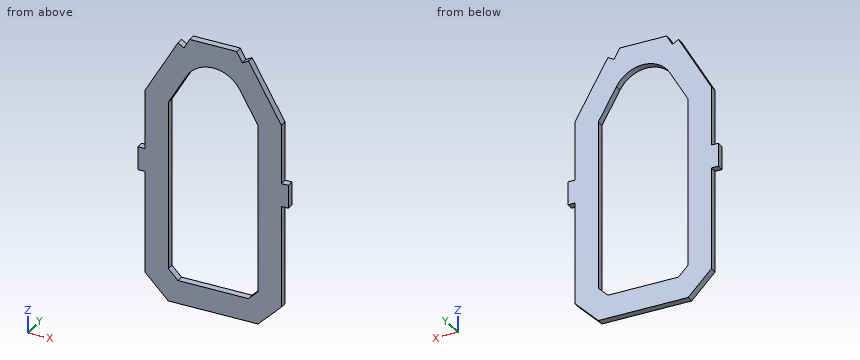
from build123d import *

# Parameters (mm, degrees)
F1_DEPTH = 1.5


with BuildPart() as f1:
    # F0 (on Front) → F1 (new body, symmetric)
    with BuildSketch(Plane.XZ):
        Polygon((-19.25, -59), (19.25, -59), (29.25, -49), (29.25, -5), (32.25, -5), (32.25, 5), (29.25, 5), (29.25, 30.43933), (15.1342262987, 54.8714219789), (12.5366059283, 53.370632716), (10.0352904902, 57.7), (-10.0352904902, 57.7), (-12.5366059283, 53.370632716), (-15.1342262987, 54.8714219789), (-29.25, 30.43933), (-29.25, 5), (-32.25, 5), (-32.25, -5), (-29.25, -5), (-29.25, -49), align=None)
        with BuildLine():
            Line((19.25, 0), (19.25, -44.8578643763))
            Line((19.25, -44.8578643763), (15.1078643763, -49))
            Line((15.1078643763, -49), (-15.1078643763, -49))
            Line((-15.1078643763, -49), (-19.25, -44.8578643763))
            Line((-19.25, -44.8578643763), (-19.25, 0))
            Line((-19.25, 0), (-19.25, 27.7582098748))
            Line((-19.25, 27.7582098748), (-11.4781226068, 41.2100565349))
            ThreePointArc((-11.4781226068, 41.2100565349), (-0.0096357275, 47.8457480828), (11.4684858529, 41.2267361773))
            Line((11.4684858529, 41.2267361773), (19.25, 27.7582098748))
            Line((19.25, 27.7582098748), (19.25, 0))
        make_face(mode=Mode.SUBTRACT)
    extrude(amount=F1_DEPTH, both=True)


solid = f1.part
Source: CAD feature listing. Evaluate the final solid. Frame: model axes, mm. Give positions to 0.01 mm unless a question says otherwise; leave off trailing zeros. Order: outer loops, then holes, each group sorted by start corner. A loop starts at its lowest first (then second) coordinate and runs counter-clockwise, first axis right, second up. Notation, with made-up numbers: (-24, 76) -> (-3, 76) arc R33 cw to (-3, 112) -> close; hole circle Ø8 at (-32.75, 61.5). An arc over 180 degrees is marked (long way). Write item = value, one per line.
Q1. Cut plane B-B, the plane x = -16.5. Output: boundary loops of the cut face in (y, z), and give its area (3 significant figures).
Data:
outline = (-1.5, -59) -> (1.5, -59) -> (1.5, -47.61) -> (-1.5, -47.61) -> close; (-1.5, 32.52) -> (1.5, 32.52) -> (1.5, 52.51) -> (-1.5, 52.51) -> close
area = 94.1 mm^2
Q2. Cut plane D-D, the plane x = -25.5. Output: boundary loops of the cut face in (y, z), and give its area (3 significant figures).
Data:
outline = (-1.5, -52.75) -> (1.5, -52.75) -> (1.5, 36.93) -> (-1.5, 36.93) -> close
area = 269 mm^2
Q3. Material intervals for line 1 (X direction, y = -0.95, z = -30.5); line 2 (Z direction, x = 4.5, y = -1.25); line 3 (Z direction, x = 29.5, y = -1), sorted ascending. Write a range as from..to.
Data:
line_1 = -29.25..-19.25, 19.25..29.25
line_2 = -59..-49, 47.06..57.7
line_3 = -5..5
Q4. Pin query (flat end, axial travel): pin 1 (1.5 mm diameter, centred on y = -0.5, z = 21.5, fed in from -X); pin 2 (1.5 mm diameter, centred on x = 30.5, y = -0.5, fed in from +Z); pin 3 (1.5 mm diameter, centred on x = 30.5, y = -0.5, fed in from -Z). Return the tip coordinate at first contact, or that it passes through.
Data:
pin_1 = -29.25
pin_2 = 5
pin_3 = -5
Q5. Cut plane C-C, the plane y = 0.3. Output: boundary loops of the cut face in (x, z) (3 decimals).
Data:
outline = (-32.25, -5) -> (-29.25, -5) -> (-29.25, -49) -> (-19.25, -59) -> (19.25, -59) -> (29.25, -49) -> (29.25, -5) -> (32.25, -5) -> (32.25, 5) -> (29.25, 5) -> (29.25, 30.439) -> (15.134, 54.871) -> (12.537, 53.371) -> (10.035, 57.7) -> (-10.035, 57.7) -> (-12.537, 53.371) -> (-15.134, 54.871) -> (-29.25, 30.439) -> (-29.25, 5) -> (-32.25, 5) -> close; hole (-19.25, -44.858) -> (-15.108, -49) -> (15.108, -49) -> (19.25, -44.858) -> (19.25, 27.758) -> (11.468, 41.227) arc R13.245 ccw to (-11.478, 41.21) -> (-19.25, 27.758) -> close
Q6. Cut plane A-A, the plane z = 25.5. Output: boundary loops of the cut face in (x, y).
Data:
outline = (-29.25, -1.5) -> (-19.25, -1.5) -> (-19.25, 1.5) -> (-29.25, 1.5) -> close; (19.25, -1.5) -> (29.25, -1.5) -> (29.25, 1.5) -> (19.25, 1.5) -> close
